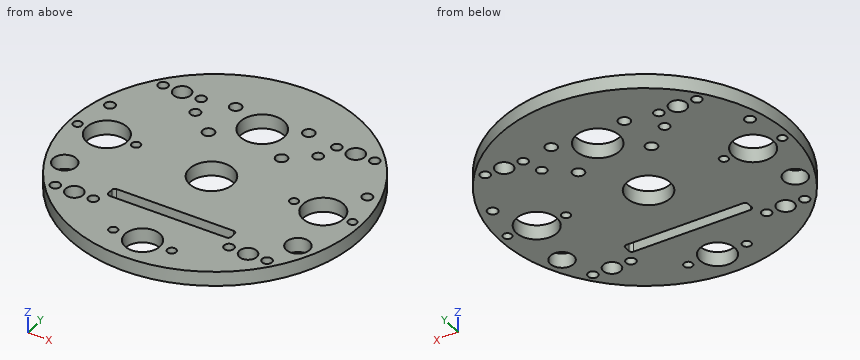
```python
from build123d import *

# Parameters (mm, degrees)
SKETCH1_R                  = 50
BOSS_EXTRUDE1_DEPTH        = 5
F_14_0_14_DIAMETER_HOLE1_D = 14
SKETCH9_R                  = 7.5
CUT_EXTRUDE1_DEPTH         = 10
SKETCH10_R                 = 2
CUT_EXTRUDE2_DEPTH         = 10
SKETCH11_R                 = 7.5
CUT_EXTRUDE3_DEPTH         = 10
SKETCH12_R                 = 3
CUT_EXTRUDE4_DEPTH         = 10
CIRPATTERN1_COUNT          = 4
SKETCH13_R                 = 1.5
SKETCH13_R_2               = 6
CUT_EXTRUDE5_DEPTH         = 10
SKETCH14_R                 = 1.75
CUT_EXTRUDE6_DEPTH         = 10
SKETCH15_R                 = 4
CUT_EXTRUDE7_DEPTH         = 10
CUT_EXTRUDE8_DEPTH         = 10
M3_CLEARANCE_HOLE1_D       = 3.4
MIRROR3_COPY_1_D           = 3.4


with BuildPart() as part:
    # Sketch1 → Boss-Extrude1 (new body)
    with BuildSketch(Plane.XY):
        Circle(SKETCH1_R)
    extrude(amount=BOSS_EXTRUDE1_DEPTH)

    # Ø14.0 (14) Diameter Hole1 (through all)
    with Locations(Plane(origin=(0, 0, 0), x_dir=(-1, 0, 0), z_dir=(0, 0, -1))):
        with Locations((37, 0), (-37, 0)):
            Hole(F_14_0_14_DIAMETER_HOLE1_D / 2)

    # Sketch9 → Cut-Extrude1 (cut)
    with BuildSketch(Plane.XY.offset(5)):
        with Locations((0, 26)):
            Circle(SKETCH9_R)
    extrude(amount=-CUT_EXTRUDE1_DEPTH, mode=Mode.SUBTRACT)

    # Sketch10 → Cut-Extrude2 (cut)
    with BuildSketch(Plane.XY.offset(5)):
        with Locations((-12.5, 31.5)):
            Circle(SKETCH10_R)
        with Locations((-12.5, 16.5)):
            Circle(SKETCH10_R)
        with Locations((12.5, 31.5)):
            Circle(SKETCH10_R)
        with Locations((12.5, 16.5)):
            Circle(SKETCH10_R)
    extrude(amount=-CUT_EXTRUDE2_DEPTH, mode=Mode.SUBTRACT)

    # Sketch11 → Cut-Extrude3 (cut)
    with BuildSketch(Plane.XY.offset(5)):
        with Locations((0, -2)):
            Circle(SKETCH11_R)
    extrude(amount=-CUT_EXTRUDE3_DEPTH, mode=Mode.SUBTRACT)

    # Sketch12 → Cut-Extrude4 (cut)
    with BuildSketch(Plane.XY.offset(5)):
        with Locations((-29.69848481, 29.69848481)):
            Circle(SKETCH12_R)
    cut_extrude4 = extrude(amount=-CUT_EXTRUDE4_DEPTH, mode=Mode.SUBTRACT)

    # CirPattern1: Cut-Extrude4 ×4 about axis
    cirpattern1_axis = Axis((0, 0, 0), (0, 0, 1))
    for i in range(1, CIRPATTERN1_COUNT):
        add(cut_extrude4.rotate(cirpattern1_axis, i * 360 / CIRPATTERN1_COUNT), mode=Mode.SUBTRACT)

    # Sketch13 → Cut-Extrude5 (cut)
    with BuildSketch(Plane.XY.offset(5)):
        with Locations((-47, 0)):
            Circle(SKETCH13_R)
        with Locations((-27, 0)):
            Circle(SKETCH13_R)
        with Locations((27, 0)):
            Circle(SKETCH13_R)
        with Locations((47, 0)):
            Circle(SKETCH13_R)
        with Locations((10, -40)):
            Circle(SKETCH13_R)
        with Locations((-10, -40)):
            Circle(SKETCH13_R)
        with Locations((0, -40)):
            Circle(SKETCH13_R_2)
    extrude(amount=-CUT_EXTRUDE5_DEPTH, mode=Mode.SUBTRACT)

    # Sketch14 → Cut-Extrude6 (cut)
    with BuildSketch(Plane.XY.offset(5)):
        with Locations((-21, 23)):
            Circle(SKETCH14_R)
        with Locations((-44, 13)):
            Circle(SKETCH14_R)
    cut_extrude6 = extrude(amount=-CUT_EXTRUDE6_DEPTH, mode=Mode.SUBTRACT)

    # Mirror1: Cut-Extrude6 across plane
    add(cut_extrude6.mirror(Plane(origin=(0, 0, 0), x_dir=(0, 0, 1), z_dir=(1, 0, 0))), mode=Mode.SUBTRACT)

    # Sketch15 → Cut-Extrude7 (cut)
    with BuildSketch(Plane.XY.offset(5)):
        with Locations((-39.87754263, -18.595203517)):
            Circle(SKETCH15_R)
        with Locations((39.87754263, -18.595203517)):
            Circle(SKETCH15_R)
    extrude(amount=-CUT_EXTRUDE7_DEPTH, mode=Mode.SUBTRACT)

    # Sketch16 → Cut-Extrude8 (cut)
    with BuildSketch(Plane.XY.offset(5)):
        with BuildLine():
            Line((-20, -22), (20, -22))
            ThreePointArc((20, -22), (20.707106781, -22.292893219), (21, -23))
            Line((21, -23), (21, -25))
            ThreePointArc((21, -25), (20.707106781, -25.707106781), (20, -26))
            Line((20, -26), (-20, -26))
            ThreePointArc((-20, -26), (-20.707106781, -25.707106781), (-21, -25))
            Line((-21, -25), (-21, -23))
            ThreePointArc((-21, -23), (-20.707106781, -22.292893219), (-20, -22))
        make_face()
    extrude(amount=-CUT_EXTRUDE8_DEPTH, mode=Mode.SUBTRACT)

    # M3 Clearance Hole1 (through all)
    with Locations(Plane.XY.offset(5)):
        with Locations((-36.19848481, -29.69848481), (-23.19848481, -29.69848481)):
            m3_clearance_hole1 = Hole(M3_CLEARANCE_HOLE1_D / 2)

    # Mirror2: M3 Clearance Hole1 across plane
    add(m3_clearance_hole1.mirror(Plane.ZX), mode=Mode.SUBTRACT)

    # Mirror3: M3 Clearance Hole1 across plane
    add(m3_clearance_hole1.mirror(Plane(origin=(0, 0, 0), x_dir=(0, 0, 1), z_dir=(1, 0, 0))), mode=Mode.SUBTRACT)

    # Mirror3 copy 1 (through all)
    with Locations(Plane(origin=(0, 0, 5), x_dir=(-1, 0, 0), z_dir=(0, 0, 1))):
        with Locations((-36.19848481, -29.69848481), (-23.19848481, -29.69848481)):
            Hole(MIRROR3_COPY_1_D / 2)


solid = part.part
```
The model under review builds one solid part; all positions refer to its coordinate system, in mm. Round coordinates to 2 decimals unless told otherwise and drop trailing zeros. Loops run counter-clockwise (first coordinate to the right, second up) from the corner with the lowest first, then second, coordinate; pieces in that order, holes last. Notation, with made-up numbers: (-13, 62.25) -> (33, 62.25) arc R29 cw to (33, 97.25) -> close; hole circle Ø6 at (37.25, 21.5). An arc over 180 degrees is marked (long way). Answer as a JSON object with one key per item and string values. Group by question number.
1) We need section A-A on x = 0. Write out the cut boundary in (y, z), then the cut area to 3 significant figures.
2) We need section C-C on x = 47. Write out the cut boundary in (y, z), then the cut area to 3 significant figures.
3) For line 1 (Y direction, x = -12.5, z = 3.15); line 2 (Y direction, x = -37.5, z = 1); line 3 (Y direction, x = 27, z = 1.1), list the stretches that pass through material, from the lowest coordinate up. Write a range as [from, to].
4) We need section B-B on y = -40. Write out the cut boundary in (x, z), then the cut area to 3 significant figures.
5) For pin 1 Ø1.5 at (y, z) = (10, 4) entering from -X, flat-tipped, find the tip position at first contact; note if it passes through.
6) We need section D-D on y = 16.5. Write out the cut boundary in (x, z), then the cut area to 3 significant figures.
Result set:
{
 "1": {"outline": "(-50, 0) -> (-46, 0) -> (-46, 5) -> (-50, 5) -> close; (-34, 0) -> (-26, 0) -> (-26, 5) -> (-34, 5) -> close; (-22, 0) -> (-9.5, 0) -> (-9.5, 5) -> (-22, 5) -> close; (5.5, 0) -> (18.5, 0) -> (18.5, 5) -> (5.5, 5) -> close; (33.5, 0) -> (50, 0) -> (50, 5) -> (33.5, 5) -> close", "area": "270 mm²"},
 "2": {"outline": "(-17.06, 0) -> (-1.5, 0) -> (-1.5, 5) -> (-17.06, 5) -> close; (1.5, 0) -> (17.06, 0) -> (17.06, 5) -> (1.5, 5) -> close", "area": "156 mm²"},
 "3": {"line 1": "[-48.41, -26], [-22, 14.5], [18.5, 29.5], [33.5, 48.41]", "line 2": "[-33.07, -30.79], [-28.6, -21.81], [-15.38, -6.98], [6.98, 28.6], [30.79, 33.07]", "line 3": "[-42.08, -31.01], [-28.39, -1.5], [1.5, 28.39], [31.01, 42.08]"},
 "4": {"outline": "(-30, 0) -> (-11.5, 0) -> (-11.5, 5) -> (-30, 5) -> close; (-8.5, 0) -> (-6, 0) -> (-6, 5) -> (-8.5, 5) -> close; (6, 0) -> (8.5, 0) -> (8.5, 5) -> (6, 5) -> close; (11.5, 0) -> (30, 0) -> (30, 5) -> (11.5, 5) -> close", "area": "210 mm²"},
 "5": {"pin 1": "x = -49.14"},
 "6": {"outline": "(-47.2, 0) -> (-14.5, 0) -> (-14.5, 5) -> (-47.2, 5) -> close; (-10.5, 0) -> (10.5, 0) -> (10.5, 5) -> (-10.5, 5) -> close; (14.5, 0) -> (47.2, 0) -> (47.2, 5) -> (14.5, 5) -> close", "area": "432 mm²"}
}
